Could you check a few things on this model? Use its own coordinates, in mm. A direction names the side the tool comes from. Round coordinates to 2 decimals unless told otherwise and drop trailing zeros. Loops run counter-clockwise (first coordinate to the right, second up) from the corner with the lowest first, then second, coordinate; pieces in that order, holes last.
from build123d import *

# Parameters (mm, degrees)
F1_DEPTH = 100
F2_W     = 30
F2_H     = 80
F3_DEPTH = 5
F5_DEPTH = 80


with BuildPart() as f1:
    # F0 (on Front) → F1 (new body)
    with BuildSketch(Plane.XZ):
        Polygon((14.5147677447, 24.9530529325), (-28.8673616138, 0.0936311307), (14.3525938692, -25.0466840632), align=None)
    extrude(amount=F1_DEPTH)

    # F2 (on face) → F3 (cut)
    with BuildSketch(Plane(origin=(-7.2573838723, 0, -12.4765264662), x_dir=(0.8643991097, 0, -0.5028063039), z_dir=(-0.5028063039, 0, -0.8643991097))):
        with Locations((0, 50)):
            Rectangle(F2_W, F2_H)
    extrude(amount=-F3_DEPTH, mode=Mode.SUBTRACT)

    # F4 (on face) → F5 (cut)
    with BuildSketch(Plane.XZ.offset(100)):
        Polygon((8.7088606468, 14.9718317595), (-17.3204169683, 0.0561786784), (8.6115563215, -15.0280104379), align=None)
    extrude(amount=-F5_DEPTH, mode=Mode.SUBTRACT)


solid = f1.part
Item 1: If I drill on line 1 along X through (y, z) = (-75.5, -3); line 2 along Z through (x, y) = (6.5, -27); line 3 along Y through (x, z) = (-2, -11), over which ranges is the centre line in solid material (lowest first)?
Results list:
line 1: x = -23.55 to -19.1, -13.6 to -12.07, 8.65 to 14.42
line 2: z = -20.48 to -18.66, -14.69 to -13.8, 13.71 to 20.36
line 3: y = -100 to -90, -10 to 0
Item 2: For faces 5 (the flat face through (-22, -49.3, -3.9)), 6 (the flat face through (-3, 0, 0)), 7 (the flat face through (-18.98, -49.44, -2.8)), 8 (the flat face through (6.948, -49.44, -17.888)), 9 (the flat face through (-2, -20, 0)), which set-ups out of +Z, -Z, +X, -X, +Y, -Y let a thin tool reach every point of the face, with its end or its side?
Results list:
face 5: -Z, -X, +Y, -Y
face 6: +Z, -Z, +X, -X, +Y
face 7: -Z
face 8: -X
face 9: -Y
Item 3: If we section it at D-D, the plane x = -7: Please give me the cut outline in (y, z).
Results list:
outline: (-100, -12.63) - (-90, -12.63) - (-90, -6.84) - (-10, -6.84) - (-10, -12.63) - (0, -12.63) - (0, 12.62) - (-100, 12.62) - (-100, 5.97) - (-20, 5.97) - (-20, -5.95) - (-100, -5.95) - close
Item 4: We'd pull the mould along Z, two halves only. Please class faces 1 (the flat face through (9, -100, 0)), 2 (the flat face through (-4.5, -60.6, -7.4)), 3 (the flat face through (-6.87, -49.3, 12.7)), 4 (the flat face through (-4.12, -60.56, 7.62)): released by +Z, released by -Z, zero draft, split by the parting line, or undercut.
Results list:
face 1: zero draft
face 2: undercut
face 3: released by +Z
face 4: undercut
Item 5: If we section it at C-C, the plane z = -17.5: Please give me the cut outline in (x, y), then the cut area to 3 significant figures.
Results list:
outline: (1.38, -100) - (14.38, -100) - (14.38, 0) - (1.38, 0) - (1.38, -10) - (7.17, -10) - (7.17, -90) - (1.38, -90) - close
area: 836 mm2
Item 6: Will these pins go through, and if not, where does the flat tip stop? pin 1 (1 mm diameter, centred on y = -70.5, z = 9, fed in from +X); pin 2 (6 mm diameter, centred on x = 4.5, y = -14.5, fed in from +Z); pin 3 (4 mm diameter, centred on x = -13, y = -73.5, fed in from -Z).
Results list:
pin 1: stops at x = 14.46
pin 2: stops at z = 20.93
pin 3: stops at z = -4.52
Item 7: If we section it at A-A, the plane y = -83.5: Please give me the cut outline in (x, z), then the cut area to 3 significant figures.
Results list:
outline: (-28.87, 0.09) - (-20.22, -4.93) - (-17.71, -0.61) - (8.22, -15.7) - (5.71, -20.02) - (14.35, -25.05) - (14.51, 24.95) - close; hole (-17.32, 0.06) - (8.61, -15.03) - (8.71, 14.97) - close
area: 543 mm2
Item 8: If we section it at B-B, the plane z = -3.5: Please give me the cut outline in (x, y), then the cut area to 3 significant figures.
Results list:
outline: (-22.69, -100) - (-11.21, -100) - (-11.21, -20) - (8.65, -20) - (8.65, -100) - (14.42, -100) - (14.42, 0) - (-22.69, 0) - close; hole (-19.39, -90) - (-12.75, -90) - (-12.75, -10) - (-19.39, -10) - close
area: 1,590 mm2
